from build123d import *

# Parameters (mm, degrees)
SKETCH1_R               = 8.213367202
TOOTHOD_DEPTH           = 6.35
TOOTHPROFILE_DEPTH      = 7.35
TOOTHPATTERN_COUNT      = 18
SKETCH7_R               = 1.5625
BORE_DEPTH              = 8.62
BORE_DEPTH_BACK         = 8.62
SKETCH11_W              = 19.982734404
SKETCH11_H              = 1.27
CUT_EXTRUDE2_DEPTH      = 10.991367202
CUT_EXTRUDE2_DEPTH_BACK = 10.991367202


with BuildPart() as part:
    # Sketch1 → ToothOD (new body, symmetric)
    with BuildSketch(Plane(origin=(0, 0, 0), x_dir=(1, 0, 0), z_dir=(0, 1, 0))):
        Circle(SKETCH1_R)
    extrude(amount=TOOTHOD_DEPTH, both=True)

    # Sketch2 → ToothProfile (cut, symmetric)
    with BuildSketch(Plane(origin=(0, 0, 0), x_dir=(1, 0, 0), z_dir=(0, 1, 0))):
        with BuildLine():
            ThreePointArc((-0.937033068, 7.763429198), (-0.590385173, 7.245254588), (0, 7.044967202))
            ThreePointArc((0, 7.044967202), (0.590385173, 7.245254588), (0.937033068, 7.763429198))
            ThreePointArc((0.937033068, 7.763429198), (0.971699064, 7.88954066), (1.007805813, 8.015247202))
            ThreePointArc((1.007805813, 8.015247202), (1.037242296, 8.083128985), (1.082411127, 8.141731201))
            ThreePointArc((1.082411127, 8.141731201), (0, 8.213367202), (-1.082411127, 8.141731201))
            ThreePointArc((-1.082411127, 8.141731201), (-1.037242296, 8.083128985), (-1.007805813, 8.015247202))
            ThreePointArc((-1.007805813, 8.015247202), (-0.971699064, 7.88954066), (-0.937033068, 7.763429198))
        make_face()
    toothprofile = extrude(amount=TOOTHPROFILE_DEPTH, both=True, mode=Mode.SUBTRACT)

    # ToothPattern: ToothProfile ×18 about axis
    toothpattern_axis = Axis((0, 0, 0), (0, 1, 0))
    for i in range(1, TOOTHPATTERN_COUNT):
        add(toothprofile.rotate(toothpattern_axis, i * 360 / TOOTHPATTERN_COUNT), mode=Mode.SUBTRACT)

    # Sketch4 → Flange (revolve)
    with BuildSketch(Plane.XY):
        with BuildLine():
            Line((0, -6.35), (8.467367202, -6.35))
            ThreePointArc((8.467367202, -6.35), (8.697013823, -6.385951298), (8.92243953, -6.442637424))
            ThreePointArc((8.92243953, -6.442637424), (9.490168107, -6.724197125), (9.991367202, -7.112))
            Line((9.991367202, -7.112), (9.991367202, -7.62))
            Line((9.991367202, -7.62), (0, -7.62))
            Line((0, -7.62), (0, -6.35))
        make_face()
        with BuildLine():
            Line((9.991367202, 7.62), (9.991367202, 7.112))
            ThreePointArc((9.991367202, 7.112), (9.490168107, 6.724197125), (8.92243953, 6.442637424))
            ThreePointArc((8.92243953, 6.442637424), (8.697013823, 6.385951298), (8.467367202, 6.35))
            Line((8.467367202, 6.35), (0, 6.35))
            Line((0, 6.35), (0, 7.62))
            Line((0, 7.62), (9.991367202, 7.62))
        make_face()
    revolve(axis=Axis((0, 8.73125, 0), (0, -1, 0)))

    # Sketch7 → Bore (cut, two sides)
    with BuildSketch(Plane.XZ) as bore_sk:
        Circle(SKETCH7_R)
    extrude(amount=BORE_DEPTH, mode=Mode.SUBTRACT)
    extrude(bore_sk.sketch, amount=-BORE_DEPTH_BACK, mode=Mode.SUBTRACT)

    # Sketch11 → Cut-Extrude2 (cut, two sides)
    with BuildSketch(Plane.XY) as cut_extrude2_sk:
        with Locations((0, 6.985)):
            Rectangle(SKETCH11_W, SKETCH11_H)
        with Locations((0, -6.985)):
            Rectangle(SKETCH11_W, SKETCH11_H)
    extrude(amount=CUT_EXTRUDE2_DEPTH, mode=Mode.SUBTRACT)
    extrude(cut_extrude2_sk.sketch, amount=-CUT_EXTRUDE2_DEPTH_BACK, mode=Mode.SUBTRACT)


solid = part.part
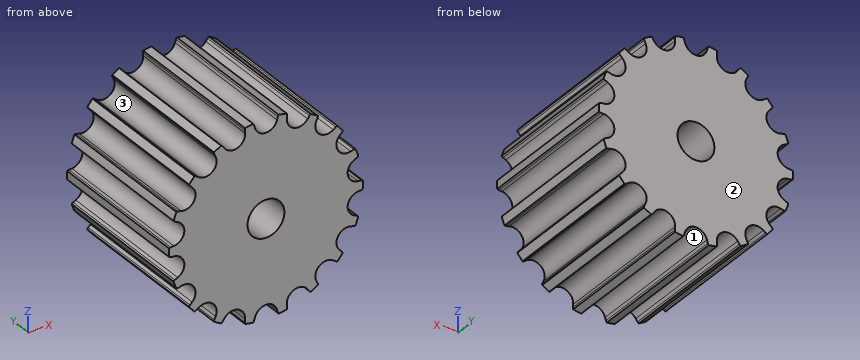
Could you check a few things on this model? Use its own coordinates, in mm. Face numbers are marked on the shaded views. Round coordinates to 2 decimals unless told otherwise and drop trailing zeros. Write each loop counter-clockwise with the first axis right and the second up, starting at its lowest first coordinate (ties: lowest second). Pieces come first, ordered by that corner, then holes. Notation, with made-up numbers: (3.25, 57.5) - (49.25, 57.5) arc R15 cw to (49.25, 71.5) - close; hole circle Ø10 at (6.25, 36.25). An arc over 180 degrees is marked (long way). Put each result on its own line as item: value. Start each with the question number.
(1) I want a section at B-B, the plane z = 0. Please give me the cut outline in (x, y).
(2) I want a section at A-A, the plane x = 0. Please give me the cut outline in (y, z).
(3) I want a section at C-C, the plane x = 3.25. Please give me the cut outline in (y, z), plus the area to 3 significant figures.
(4) I need wall thicknesses on probe 1 along X at (y, z) = (3.5, 0); probe 2 along X at (y, z) = (-4.5, -1.25); probe 3 along X at (y, z) = (1, 5.5). Which ranges of each line are inside material? Lowest first, please.
(5) Thinking about a two-plate mould opening in Z: for the marked faces 1, 2 and 3, which applies, released by +Z, released by -Z, zero draft, split by the parting line, or undercut?
Here are the results:
1. outline: (-8.21, -6.35) - (-1.56, -6.35) - (-1.56, 6.35) - (-8.21, 6.35) - close; (1.56, -6.35) - (8.21, -6.35) - (8.21, 6.35) - (1.56, 6.35) - close
2. outline: (-6.35, -7.04) - (6.35, -7.04) - (6.35, -1.56) - (-6.35, -1.56) - close; (-6.35, 1.56) - (6.35, 1.56) - (6.35, 7.04) - (-6.35, 7.04) - close
3. outline: (-6.35, -6.71) - (6.35, -6.71) - (6.35, 6.71) - (-6.35, 6.71) - close
3. area: 170 mm^2
4. probe 1: x = -8.21 to -1.56, 1.56 to 8.21
4. probe 2: x = -6.93 to -0.94, 0.94 to 6.93
4. probe 3: x = -6.1 to -5.94, -4.42 to 4.42, 5.94 to 6.1
5. face 1: released by -Z
5. face 2: zero draft
5. face 3: undercut
